Model file for the job. Use its own axes, mm. A direction names the side the tool comes from. Coordinates: 2 decimals unless noted, no trailing zeros. Write each loop counter-clockwise with the first axis right and the second up, starting at its lowest first coordinate (ties: lowest second). Pieces come first, ordered by that corner, then holes. Notation, with made-up numbers: M 55,13.5 L 61,13.5 A19 cw 61,43.5 Z; hole C -27,45 d8. An arc over 180 degrees is marked long. One line per question, with ' | ' between items. Start each with the question number.
(1) Flat gauge pins, fed straight in: pin 1 Ø6 at (y, z) = (15, -8.5) entering from -X; pin 2 Ø1 at (x, z) = (-7.5, 1) entering from +Y; pin 3 Ø12 at (x, y) = (6, 26) entering from +Z. Where does each tip first touch, or does it go through?
(2) Cut at A-A (y = 20). Write the cut outline in (x, z).
(3) Wall check: probe 1 along Y at (x, z) = (-1.5, -9); probe 2 along X at (y, z) = (48, 2.5); probe 3 along X at (y, z) = (12, -2.5). Give the ranges that are in metal, low to high.
(4) Tool access for faces 1 (the face through (1.855, 48.253, -0.151)), 2 (the face through (1.38, 23.86, -6.2)), 3 (the face through (0, 0, 0)): list every direction of +Z, -Z, +X, -X, +Y, -Y with a clear straight run to the whole face (end or side of a thin tool).
(5) Two-plate mould, pull along X, no slides. Class faces 4 (the face through (-1.867, 48.298, -0.151)), 5 (the face through (6, 43.18, 3)), 6 (the face through (0.45, 0.81, -2.03)): +X half, -X half, draft (parallel to the pull), parting line (faces both ways), or undercut.
from build123d import *

# Parameters (mm, degrees)
CHAMFER4_SIZE           = 5.08
CUT_EXTRUDE2_DEPTH      = 13.517807
CUT_EXTRUDE2_DEPTH_BACK = 13.517807


with BuildPart() as part:
    # Sketch1 one side → Revolve13 (revolve)
    with BuildSketch(Plane.XY):
        Polygon((-6.35, 43.18), (-6.35, 0), (0, 0), (0, 45.72), (-12.517807, 45.72), (-12.517807, 43.18), align=None)
        with BuildLine():
            ThreePointArc((0, 50.41009), (-6.683794, 49.199075), (-12.517807, 45.72))
            Line((-12.517807, 45.72), (0, 45.72))
            Line((0, 45.72), (0, 50.41009))
        make_face()
    revolve(axis=Axis((0, -10.13615, 0), (0, 1, 0)))

    # Chamfer4
    chamfer4_edges = [part.edges().sort_by_distance(p)[0] for p in [
        (6.35, 0, 0),
    ]]
    chamfer(chamfer4_edges, length=CHAMFER4_SIZE)

    # Sketch4 → Cut-Extrude2 (cut, two sides)
    with BuildSketch(Plane.XY) as cut_extrude2_sk:
        Polygon((-32.117638, 161.194555), (-2.39261, 50.259241), (-1.522582, 47.012254), (1.522582, 47.012254), (2.39261, 50.259241), (32.117638, 161.194555), (32.117638, 390.891931), (-32.117638, 390.891931), align=None)
    extrude(amount=CUT_EXTRUDE2_DEPTH, mode=Mode.SUBTRACT)
    extrude(cut_extrude2_sk.sketch, amount=-CUT_EXTRUDE2_DEPTH_BACK, mode=Mode.SUBTRACT)


solid = part.part
Filled in:
1) pin 1: x = -3.17 | pin 2: y = 49.05 | pin 3: z = 6.35
2) outline: C 0,0 d12.7
3) probe 1: 43.18 to 47.01 | probe 2: -8.93 to -1.79, 1.79 to 8.93 | probe 3: -5.84 to 5.84
4) face 1: +Z, -Z, +Y | face 2: -Y | face 3: +Z, -Z, +X, -X, -Y
5) face 4: undercut | face 5: draft | face 6: parting line
